The figure shows three views and two pictorial views of one solid part (mm, origin at its lowest corner). Answer the questions. A direction names the side the tool comes from. Coordinates: 2 decimals unless noted, no trailing zeros. Write each loop counter-clockwise with the first axis right and the second up, starting at its lowest first coordinate (ties: lowest second). Pieces come first, ordered by that corner, then holes. Notation, with made-up numbers: (2, 34.5) - (26, 34.5) arc R29 ccw to (26, 65.5) - close; hole circle Ø3 at (72, 15). An arc over 180 degrees is marked (long way). Use a Markdown table: item, result. Add a question column.
(1) A tool of negligible diameter and unlimited length cuts with its end or side. For the marked faces 4, 5 and 6, from which of +Z, -Z, +X, -X, +Y, -Y can it reach the whole face along a straight path? Write none if from no direction.
(2) The part is cut by section C-C, the plane y = 12.7. Give the vertices of the cut face in (x, z).
(3) For a pull along X with two mould halves and no side action, classify the marked faces 1, 2 and 3 as released by +X, released by -X, zero draft, split by the parting line, or undercut.
(4) The part is cut by section A-A, the plane x = 12.7. Give the vertices of the cut face in (y, z).
(5) Given pin 1 Ø4 at (x, z) = (50, 5.5) entering from -Y; pin 2 Ø3 at (x, z) = (50, 10.5) entering from +Y; pin 3 Ø4 at (y, z) = (52, 9) entering from -X, each flat-ended and moving along its own axis, determine where each tip first touches the part or whether it passes through.
(6) Find the intervals of material crossed by line 1 (X direction, y = 11.5, z = 3.75); line 2 (X direction, y = 21, z = 3.5); line 3 (Y direction, x = 23, z = 3), in increasing order. Write a range as from..to.
(7) The part is cut by section D-D, the plane z = 7. State how many separate pieces and enclosed holes the cut face has, then the cut area to 3 significant figures.
(8) The part is cut by section B-B, the plane y = 5.5. Give the vertices of the cut face in (x, z).
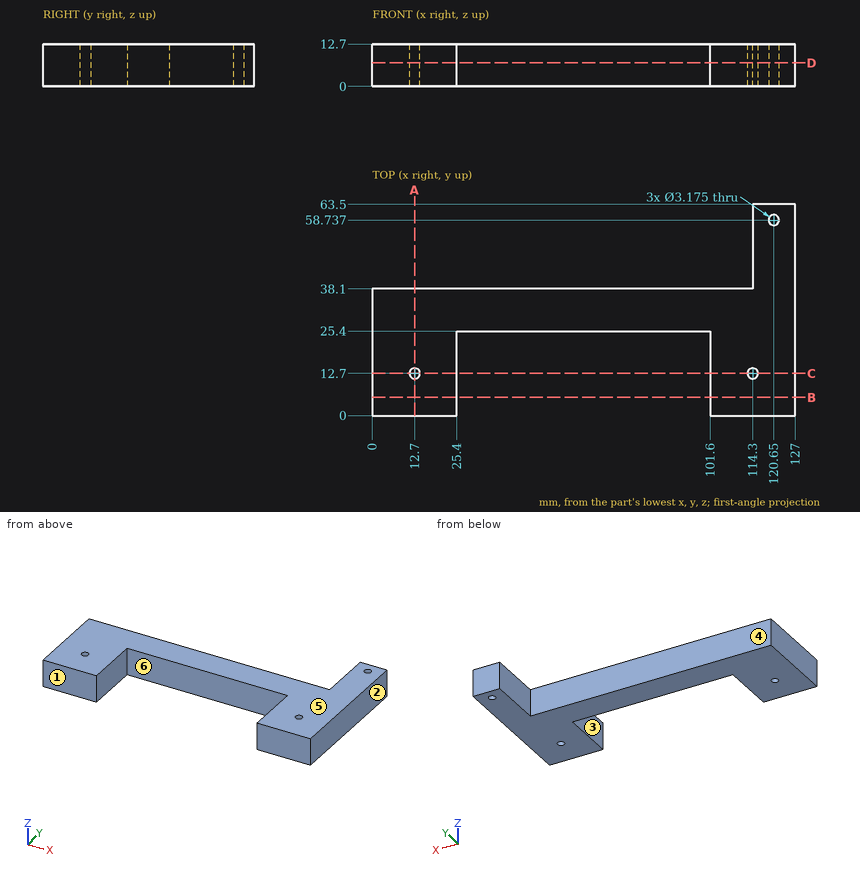
Model answer:
| question | item | result |
|---|---|---|
| 1 | face 4 | +Z, -Z, -X, +Y |
| 1 | face 5 | +Z, +X, -X, +Y, -Y |
| 1 | face 6 | +Z, -Z, -Y |
| 2 | outline | (0, 0) - (11.11, 0) - (11.11, 12.7) - (0, 12.7) - close; (14.29, 0) - (25.4, 0) - (25.4, 12.7) - (14.29, 12.7) - close; (101.6, 0) - (112.71, 0) - (112.71, 12.7) - (101.6, 12.7) - close; (115.89, 0) - (127, 0) - (127, 12.7) - (115.89, 12.7) - close |
| 3 | face 1 | zero draft |
| 3 | face 2 | released by +X |
| 3 | face 3 | undercut |
| 4 | outline | (0, 0) - (11.11, 0) - (11.11, 12.7) - (0, 12.7) - close; (14.29, 0) - (38.1, 0) - (38.1, 12.7) - (14.29, 12.7) - close |
| 5 | pin 1 | y = 25.4 |
| 5 | pin 2 | y = 38.1 |
| 5 | pin 3 | x = 114.3 |
| 6 | line 1 | 0..11.66, 13.74..25.4, 101.6..113.26, 115.34..127 |
| 6 | line 2 | 0..25.4, 101.6..127 |
| 6 | line 3 | 0..38.1 |
| 7 | separate pieces | 1 |
| 7 | enclosed holes | 3 |
| 7 | area | 3,200 mm^2 |
| 8 | outline | (0, 0) - (25.4, 0) - (25.4, 12.7) - (0, 12.7) - close; (101.6, 0) - (127, 0) - (127, 12.7) - (101.6, 12.7) - close |
